```python
from build123d import *

# Parameters (mm, degrees)
F2_DEPTH = 20


with BuildPart() as f2:
    # F1 (on Front) → F2 (new body)
    with BuildSketch(Plane.XZ):
        with BuildLine():
            Line((-130, 20), (-130, 0))
            Line((-130, 0), (130, 0))
            Line((130, 0), (130, 20))
            Line((130, 20), (100, 20))
            Line((100, 20), (41.711543, 145))
            Line((41.711543, 145), (27, 145))
            Line((27, 145), (27, 135))
            ThreePointArc((27, 135), (0, 108), (-27, 135))
            Line((-27, 135), (-27, 145))
            Line((-27, 145), (-41.711543, 145))
            Line((-41.711543, 145), (-100, 20))
            Line((-100, 20), (-130, 20))
        make_face()
        Polygon((66.898662, 20), (-66.898662, 20), (-39.852818, 78), (39.852818, 78), align=None, mode=Mode.SUBTRACT)
    extrude(amount=F2_DEPTH)


solid = f2.part
```
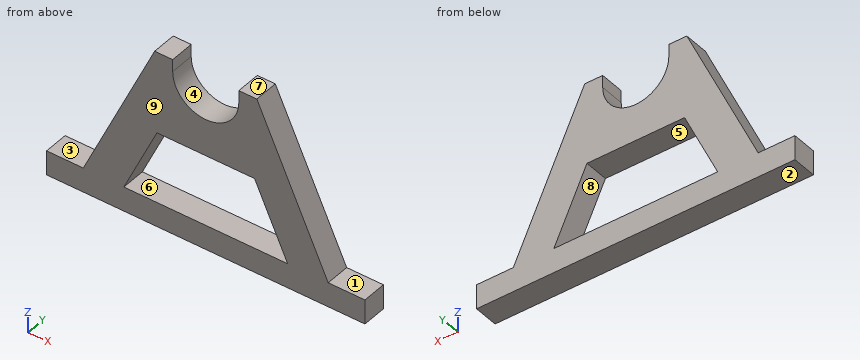
Geometry check sheet. Reference: the model listing, model coordinates, mm. Face numbers are marked on the shaded views. A direction names the side the tool comes from. Round coordinates to 2 decimals unless told otherwise and drop trailing zeros. Loops run counter-clockwise (first coordinate to the right, second up) from the corner with the lowest first, then second, coordinate; pieces in that order, holes last. Notation, with made-up numbers: (23, -31.75) - (59, -31.75) arc R8 ccw to (59, -22.75) - close; hole circle Ø9 at (44, 83.25). An arc over 180 degrees is marked (long way). Use a Markdown table: item, result.
Q1. Material ranges on line 1 (Z direction, x = 114.5, y = -16); line 2 (X direction, y = -5.75, z = 59.5); line 3 (Z direction, x = -58.5, y = -4.5), recorded low to high.
Solutions:
| item | result |
|---|---|
| line 1 | z = 0 to 20 |
| line 2 | x = -81.58 to -48.48, 48.48 to 81.58 |
| line 3 | z = 0 to 20, 38.01 to 109 |
Q2. Cross-section at B-B on z = 131. Record the cut outline in (x, y).
Solutions:
| item | result |
|---|---|
| outline | (-48.24, -20) - (-26.7, -20) - (-26.7, 0) - (-48.24, 0) - close; (26.7, -20) - (48.24, -20) - (48.24, 0) - (26.7, 0) - close |
Q3. Cross-section at D-D on z = 85. Record the cut outline in (x, y), plus the area to 3 significant figures.
Solutions:
| item | result |
|---|---|
| outline | (-69.69, -20) - (69.69, -20) - (69.69, 0) - (-69.69, 0) - close |
| area | 2,790 mm2 |
Q4. Draft check along Z on the marked faces 6, 7, 8 and 9. Enter one of: released by +Z, released by -Z, zero draft, split by the parting line, or undercut.
Solutions:
| item | result |
|---|---|
| face 6 | undercut |
| face 7 | released by +Z |
| face 8 | undercut |
| face 9 | zero draft |
Q5. Cross-section at A-A on x = 0. Record the cut outline in (y, z), plus the area to 3 significant figures.
Solutions:
| item | result |
|---|---|
| outline | (-20, 0) - (0, 0) - (0, 20) - (-20, 20) - close; (-20, 78) - (0, 78) - (0, 108) - (-20, 108) - close |
| area | 1,000 mm2 |
Q6. Access from +Z, -Z, +X, -X, +Y, -Y to the whole of each face (thin tool, end or side, straight path). Record for the marked faces 1, 2, 3, 4 and 5.
Solutions:
| item | result |
|---|---|
| face 1 | +Z, +X, +Y, -Y |
| face 2 | -Z, +X, -X, +Y, -Y |
| face 3 | +Z, -X, +Y, -Y |
| face 4 | +Z, +Y, -Y |
| face 5 | +Y, -Y |
Q7. Go/stop test with flat-tipped pins: P1, Ø10, axis at x = -118.5, y = -7, coming from the +Z side; P2, Ø3, axis at y = -9.5, z = 97, coming from the -X side; P3, Ø3, axis at y = -6, z = 138, coming from the -X side. Record where each tip stops, or that it passes through.
Solutions:
| item | result |
|---|---|
| P1 | stops at z = 20 |
| P2 | stops at x = -64.79 |
| P3 | stops at x = -45.68 |
Q8. Cross-section at C-C on y = -5.75. Record the cut outline in (x, z), plus the area to 3 significant figures.
Solutions:
| item | result |
|---|---|
| outline | (-130, 0) - (130, 0) - (130, 20) - (100, 20) - (41.71, 145) - (27, 145) - (27, 135) arc R27 cw to (-27, 135) - (-27, 145) - (-41.71, 145) - (-100, 20) - (-130, 20) - close; hole (-66.9, 20) - (66.9, 20) - (39.85, 78) - (-39.85, 78) - close |
| area | 15,000 mm2 |
